For this review, take the finished solid that the model builds, in its own axes (mm). Face numbers are marked on the shaded views. A direction names the side the tool comes from. Give positions to 0.01 mm unless a question says otherwise; leave off trailing zeros. Write each loop counter-clockwise with the first axis right and the second up, starting at its lowest first coordinate (ties: lowest second). Pieces come first, ordered by that corner, then holes. Notation, with made-up numbers: M 13.25,87 L 24.25,87 A28 ccw 24.25,119 Z; hole C -24,3 d2. An arc over 180 degrees is marked long. One line per item, written item: value. Start each with the question number.
Item 1: Tool access review of the marked faces 3, 4 and 5: name each direction out of +Z, -Z, +X, -X, +Y, -Y from which nothing blocks a thin tool from reaching the whole face with its end or side.
Item 2: To check wall thickness, follow probe 1 along Y at (x, z) = (2, 0); probe 2 along Z at (x, y) = (2, -4); probe 3 along X at (y, z) = (3, 12). State the ranges of each line that lie inside material, in increasing order.
Item 3: Consider section A-A, the plane x = 7. Write out the cut boundary in (y, z), and give its area (3 significant figures).
Item 4: Consider section C-C, the plane z = 0. Write out the cut boundary in (x, y).
Item 5: Consider section B-B, the plane y = 0. Write out the cut boundary in (x, z), and give its area (3 significant figures).
Item 6: Clearance check with flat-ended pins moving along their axes: pin 1 Ø1.5 at (x, y) = (4, 5.5) entering from -Z; pin 2 Ø5 at (x, z) = (1, -4.5) entering from -Y; pin 3 Ø4 at (x, z) = (7.5, 9) entering from -Y. State where each tip first meets the part, or that it passes through.
Item 7: Mouldability with a two-part tool opening along Z and no side actions: class the marked faces 1 and 2 as released by +Z, released by -Z, zero draft, split by the parting line, or undercut.
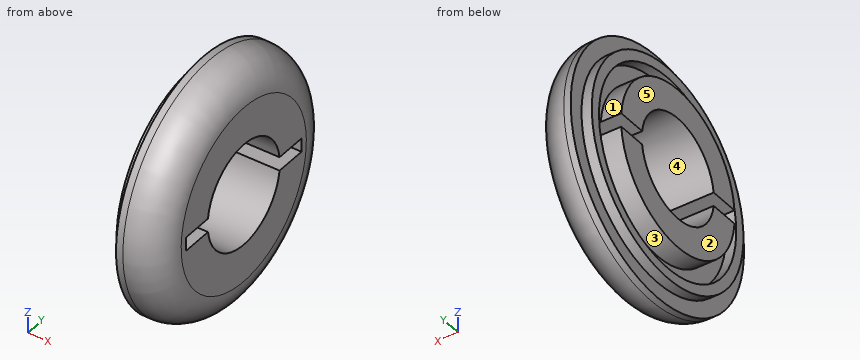
```python
from build123d import *

# Parameters (mm, degrees)
F2_R     = 5
F4_DEPTH = 9.001


with BuildPart() as f1:
    # F0 (on Front) → F1 (revolve)
    with BuildSketch(Plane.XZ):
        Polygon((0, 11.8), (0, 7.5), (9, 7.5), (9, 18), (3, 18), (3, 15.75), (1.5, 15.75), (1.5, 14.25), (3, 14.25), (3, 11.8), align=None)
    revolve(axis=Axis((4.5, 0, 0), (1, 0, 0)))

    # F2
    f2_edges = [f1.edges().sort_by_distance(p)[0] for p in [
        (9, 0, -18),
    ]]
    fillet(f2_edges, radius=F2_R)

    # F3 (on face) → F4 (cut, through all)
    with BuildSketch(Plane.YZ.offset(9)):
        with BuildLine():
            Line((-7.433034, 1), (-12, 1))
            Line((-12, 1), (-12, -1))
            Line((-12, -1), (-7.433034, -1))
            ThreePointArc((-7.433034, -1), (-7.5, 0), (-7.433034, 1))
        make_face()
        with BuildLine():
            Line((7.433034, 1), (-7.433034, 1))
            ThreePointArc((-7.433034, 1), (-7.5, 0), (-7.433034, -1))
            Line((-7.433034, -1), (7.433034, -1))
            ThreePointArc((7.433034, -1), (7.48324, -0.50112), (7.5, 0))
            ThreePointArc((7.5, 0), (7.48324, 0.50112), (7.433034, 1))
        make_face()
        with BuildLine():
            Line((12, 1), (7.433034, 1))
            ThreePointArc((7.433034, 1), (7.48324, 0.50112), (7.5, 0))
            ThreePointArc((7.5, 0), (7.48324, -0.50112), (7.433034, -1))
            Line((7.433034, -1), (12, -1))
            Line((12, -1), (12, 1))
        make_face()
    extrude(amount=-F4_DEPTH, mode=Mode.SUBTRACT)


solid = f1.part
```
Model answer:
1. face 3: -X
1. face 4: +X, -X
1. face 5: +Z, -Z, -X, +Y, -Y
2. probe 1: y = -15.75 to -14.25, 14.25 to 15.75
2. probe 2: z = -15.23 to -13.68, -11.1 to -6.34, 6.34 to 11.1, 13.68 to 15.23
2. probe 3: x = 3 to 9
3. outline: C 0,0 d34; hole M -12,-1 L -7.43,-1 A7.5 ccw 7.43,-1 L 12,-1 L 12,1 L 7.43,1 A7.5 ccw -7.43,1 L -12,1 Z
3. area: 713 mm2
4. outline: M 1.5,-15.75 L 3,-15.75 L 3,-18 L 4,-18 A5 ccw 9,-13 L 9,-12 L 3,-12 L 3,-14.25 L 1.5,-14.25 Z; M 1.5,14.25 L 3,14.25 L 3,12 L 9,12 L 9,13 A5 ccw 4,18 L 3,18 L 3,15.75 L 1.5,15.75 Z
5. outline: M 0,-11.8 L 3,-11.8 L 3,-14.25 L 1.5,-14.25 L 1.5,-15.75 L 3,-15.75 L 3,-18 L 4,-18 A5 ccw 9,-13 L 9,-7.5 L 0,-7.5 Z; M 0,7.5 L 9,7.5 L 9,13 A5 ccw 4,18 L 3,18 L 3,15.75 L 1.5,15.75 L 1.5,14.25 L 3,14.25 L 3,11.8 L 0,11.8 Z
5. area: 146 mm2
6. pin 1: stops at z = -17.36
6. pin 2: stops at y = -17.75
6. pin 3: stops at y = -15.82
7. face 1: undercut
7. face 2: zero draft
